Verification items for the finished model (mm, model axes). A direction names the side the tool comes from. Round coordinates to 2 decimals unless told otherwise and drop trailing zeros. Answer as a JSON object with one key per item and string values. Group by question number.
1) Thickness scan on line 1 (X direction, y = 29.5, z = 2.6); line 2 (Y direction, x = -29, z = 2.3); line 3 (Y direction, x = -23, z = 3.6). Record the ranges inside material, lowest first.
2) Section check A-A (z = 1.5). State how many separate pieces and enclosed holes the cut face has, then the cut area to 3 significant figures.
3) Set-up check for faces 1 (the cylindrical face through (-110, 0, 3)), 2 (the flat face through (25, -102.664, 3)), 3 (the flat face through (-97, 2.575, 3)): record each of +Z, -Z, +X, -X, +Y, -Y from which the full face is reachable in a straight line by a thin tool's end or side.
4) Mould release check, pull along X, two halves, no side actions. Record for faces 4 (the cylindrical face through (-55.121, -95.193, 2.539)), 5 (the cylindrical face through (10.615, -106.664, 2.539)), 6 (the flat face through (7.8, 95, 3)): +X half, -X half, draft (parallel to the pull), parting line (faces both ways), or undercut.
5) Go/stop test with flat-tipped pins: pin 1 Ø1.5 at (x, y) = (-72.5, 54.5) entering from +Z; pin 2 Ø2.5 at (x, z) = (-24, 3.5) entering from -Y; pin 3 Ø1.5 at (x, z) = (7, 2.5) entering from -Y; pin 4 Ø1.4 at (y, z) = (-36.5, 3.5) entering from -X. Record where each tip stops, or that it passes through.
```python
from build123d import *

# Parameters (mm, degrees)
MODEL_R             = 2.9
MODEL_R_2           = 3
MODEL_R_3           = 4.665
MODEL_R_4           = 1.95
MODEL_W             = 10
MODEL_H             = 5.15
MODEL_W_2           = 19.6
MODEL_H_2           = 4.75
BOSS_EXTRUDE1_DEPTH = 5.15


with BuildPart() as part:
    # Model → Boss-Extrude1 (new body)
    with BuildSketch(Plane.XY):
        with BuildLine():
            Line((-56.520735382, 77.896206612), (-95.720735382, 9.999814955))
            Line((-95.720735382, 9.999814955), (-109.544528393, 9.999814955))
            ThreePointArc((-109.544528393, 9.999814955), (-110, -0.000331846), (-109.544468057, -10.000475899))
            Line((-109.544468057, -10.000475899), (-95.72019722, -10.000475899))
            Line((-95.72019722, -10.000475899), (-56.52019722, -77.896867556))
            Line((-56.52019722, -77.896867556), (-63.432093724, -89.868623478))
            ThreePointArc((-63.432093724, -89.868623478), (-54.999779481, -95.262921733), (-46.112001713, -99.868329805))
            Line((-46.112001713, -99.868329805), (-39.2, -87.896391657))
            Line((-39.2, -87.896391657), (-7.8, -87.896391657))
            Line((-7.8, -87.896391657), (-7.8, -102.664454178))
            Line((-7.8, -102.664454178), (3.176931839, -102.664454178))
            ThreePointArc((3.176931839, -102.664454178), (10.74, -106.664454178), (18.303068161, -102.664454178))
            Line((18.303068161, -102.664454178), (32.2, -102.664454178))
            Line((32.2, -102.664454178), (32.2, -87.896391657))
            Line((32.2, -87.896391657), (39.2, -87.896391657))
            Line((39.2, -87.896391657), (46.112001713, -99.868329805))
            ThreePointArc((46.112001713, -99.868329805), (54.999874175, -95.262867061), (63.432272389, -89.86849737))
            Line((63.432272389, -89.86849737), (56.520280769, -77.896576702))
            Line((56.520280769, -77.896576702), (95.720280769, -10.000185045))
            Line((95.720280769, -10.000185045), (109.544494609, -10.000185045))
            ThreePointArc((109.544494609, -10.000185045), (109.999999999, -0.000331846), (109.544554943, 9.999524101))
            Line((109.544554943, 9.999524101), (95.720818931, 9.999524101))
            Line((95.720818931, 9.999524101), (56.520818931, 77.895915758))
            Line((56.520818931, 77.895915758), (63.432925851, 89.868036131))
            ThreePointArc((63.432925851, 89.868036131), (55.000220519, 95.262667099), (46.112001713, 99.868329805))
            Line((46.112001713, 99.868329805), (39.2, 87.896391657))
            Line((39.2, 87.896391657), (7.8, 87.896391657))
            Line((7.8, 87.896391657), (7.8, 102.664454178))
            Line((7.8, 102.664454178), (-3.176931839, 102.664454178))
            ThreePointArc((-3.176931839, 102.664454178), (-10.74, 106.664454178), (-18.303068161, 102.664454178))
            Line((-18.303068161, 102.664454178), (-32.2, 102.664454178))
            Line((-32.2, 102.664454178), (-32.2, 87.896391657))
            Line((-32.2, 87.896391657), (-39.2, 87.896391657))
            Line((-39.2, 87.896391657), (-46.112001713, 99.868329805))
            ThreePointArc((-46.112001713, 99.868329805), (-55.000125824, 95.262721771), (-63.432747187, 89.86816224))
            Line((-63.432747187, 89.86816224), (-56.520735382, 77.896206612))
        make_face()
        with Locations((-63, 0)):
            Circle(MODEL_R, mode=Mode.SUBTRACT)
        with Locations((-31.5, -54.559600438)):
            Circle(MODEL_R, mode=Mode.SUBTRACT)
        with Locations((31.5, -54.559600438)):
            Circle(MODEL_R, mode=Mode.SUBTRACT)
        with Locations((63, 0)):
            Circle(MODEL_R, mode=Mode.SUBTRACT)
        with Locations((31.5, 54.559600438)):
            Circle(MODEL_R, mode=Mode.SUBTRACT)
        with Locations((-31.5, 54.559600438)):
            Circle(MODEL_R_2, mode=Mode.SUBTRACT)
        Circle(MODEL_R_3, mode=Mode.SUBTRACT)
        with Locations((10.74, -97.514454178)):
            Circle(MODEL_R_4, mode=Mode.SUBTRACT)
        with Locations((-10.74, 97.514454177)):
            Circle(MODEL_R_4, mode=Mode.SUBTRACT)
        with Locations((79, 0)):
            Rectangle(MODEL_W, MODEL_H, mode=Mode.SUBTRACT)
        with Locations((97, 0)):
            Rectangle(MODEL_W, MODEL_H, mode=Mode.SUBTRACT)
        Polygon((34.769984585, 65.37337988), (39.230015415, 62.79837988), (44.230015415, 71.458633918), (39.769984585, 74.033633918), align=None, mode=Mode.SUBTRACT)
        Polygon((43.769984585, 80.961837148), (48.230015415, 78.386837148), (53.230015415, 87.047091186), (48.769984585, 89.622091186), align=None, mode=Mode.SUBTRACT)
        Polygon((-48.230015415, 78.386837148), (-43.769984585, 80.961837148), (-48.769984585, 89.622091186), (-53.230015415, 87.047091186), align=None, mode=Mode.SUBTRACT)
        Polygon((-39.230015415, 62.79837988), (-34.769984585, 65.37337988), (-39.769984585, 74.033633918), (-44.230015415, 71.458633918), align=None, mode=Mode.SUBTRACT)
        with Locations((-79, 0)):
            Rectangle(MODEL_W, MODEL_H, mode=Mode.SUBTRACT)
        with Locations((-97, 0)):
            Rectangle(MODEL_W, MODEL_H, mode=Mode.SUBTRACT)
        Polygon((-34.769984585, -65.37337988), (-39.230015415, -62.79837988), (-44.230015415, -71.458633918), (-39.769984585, -74.033633918), align=None, mode=Mode.SUBTRACT)
        Polygon((-43.769984585, -80.961837148), (-48.230015415, -78.386837148), (-53.230015415, -87.047091186), (-48.769984585, -89.622091186), align=None, mode=Mode.SUBTRACT)
        Polygon((39.230015415, -62.79837988), (34.769984585, -65.37337988), (39.769984585, -74.033633918), (44.230015415, -71.458633918), align=None, mode=Mode.SUBTRACT)
        Polygon((48.230015415, -78.386837148), (43.769984585, -80.961837148), (48.769984585, -89.622091186), (53.230015415, -87.047091186), align=None, mode=Mode.SUBTRACT)
        Polygon((33.357314709, 18.17343612), (29.243694041, 15.79843612), (39.043694041, -1.175661794), (43.157314709, 1.199338206), align=None, mode=Mode.SUBTRACT)
        Polygon((32.417314709, -19.80156388), (28.303694041, -17.42656388), (18.503694041, -34.400661794), (22.617314709, -36.775661794), align=None, mode=Mode.SUBTRACT)
        with Locations((-10.74, -35.6)):
            Rectangle(MODEL_W_2, MODEL_H_2, mode=Mode.SUBTRACT)
        Polygon((-33.357314709, -18.17343612), (-29.243694041, -15.79843612), (-39.043694041, 1.175661794), (-43.157314709, -1.199338206), align=None, mode=Mode.SUBTRACT)
        Polygon((-32.417314709, 19.80156388), (-28.303694041, 17.42656388), (-18.503694041, 34.400661794), (-22.617314709, 36.775661794), align=None, mode=Mode.SUBTRACT)
        Polygon((38.982587357, 20.659086443), (43.096208025, 23.034086443), (30.756208025, 44.407593408), (26.642587357, 42.032593408), align=None, mode=Mode.SUBTRACT)
        Polygon((37.382587357, -23.430367735), (41.496208025, -25.805367735), (53.836208025, -4.431860769), (49.722587357, -2.056860769), align=None, mode=Mode.SUBTRACT)
        Polygon((2.4, -44.089454178), (-1.6, -44.089454178), (-1.6, -48.839454177), (2.4, -48.839454177), (2.4, -92.939454178), (22, -92.939454178), (22, -48.839454177), (23.08, -48.839454177), (23.08, -44.089454178), (19.08, -44.089454178), (19.08, -40.139454177), (2.4, -40.139454177), align=None, mode=Mode.SUBTRACT)
        Polygon((-38.982587357, -20.659086443), (-43.096208025, -23.034086443), (-30.756208025, -44.407593408), (-26.642587357, -42.032593408), align=None, mode=Mode.SUBTRACT)
        Polygon((-37.382587357, 23.430367735), (-41.496208025, 25.805367735), (-53.836208025, 4.431860769), (-49.722587357, 2.056860769), align=None, mode=Mode.SUBTRACT)
        with Locations((10.74, 35.6)):
            Rectangle(MODEL_W_2, MODEL_H_2, mode=Mode.SUBTRACT)
        Polygon((-2.4, 44.089454178), (1.6, 44.089454178), (1.6, 48.839454177), (-2.4, 48.839454177), (-2.4, 92.939454178), (-22, 92.939454178), (-22, 48.839454177), (-23.08, 48.839454177), (-23.08, 44.089454178), (-19.08, 44.089454178), (-19.08, 40.139454177), (-2.4, 40.139454177), align=None, mode=Mode.SUBTRACT)
    extrude(amount=BOSS_EXTRUDE1_DEPTH)


solid = part.part
```
Returned:
{
 "1": {"line 1": "-84.46 to -26.82, -21.33 to 33.88, 39.36 to 84.46", "line 2": "-87.9 to -56.03, -53.09 to -43.39, -37.95 to 17.83, 25.72 to 52.9, 56.22 to 102.66", "line 3": "-87.9 to 26.61, 36.11 to 44.09, 48.84 to 102.66"},
 "2": {"separate pieces": "1", "enclosed holes": "33", "area": "25,400 mm2"},
 "3": {"face 1": "+Z, -Z, -X", "face 2": "+Z, -Z, +X, -Y", "face 3": "+Z, -Z"},
 "4": {"face 4": "-X half", "face 5": "parting line", "face 6": "undercut"},
 "5": {"pin 1": "through", "pin 2": "y = -87.9", "pin 3": "y = -106.16", "pin 4": "x = -80.82"}
}
